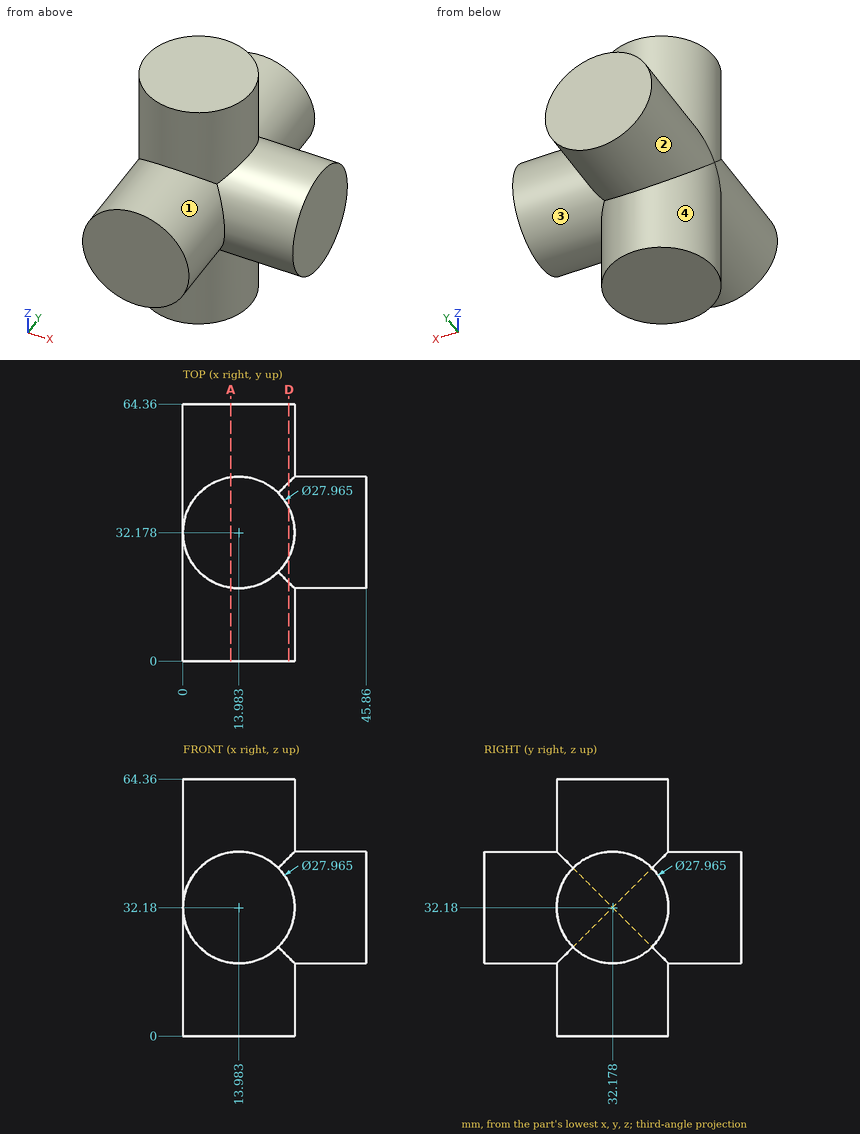
For this review, use the dimensioned drawing (mm, ordinates from the lowest corner) and the shaded views. A direction names the side the tool comes from. Give positions to 0.01 mm unless a question says otherwise; leave off trailing zeros. Order: outer loops, then holes, each group sorted by start corner. A loop starts at its lowest first (then second) coordinate and runs counter-clockwise, first axis right, second up. Notation, with made-up numbers: (78, -25) -> (85, -25) arc R20 ccw to (85, -1) -> close; hole circle Ø2 at (57, 40). An arc over 180 degrees is marked (long way). Write item = value, one per line. Start each with the question number.
(1) Take a section at A-A (x = 12). Write out the cut boundary in (y, z).
(2) For L1, parallel to Y at x = 20, z = 5 (1 decimal); L2, parallel to Z at x = 3, y = 45 (1 decimal); L3, parallel to X at y = 27, z = 27 (1 decimal), list the stretches that pass through material, from the lowest coordinate up. Write a range as from..to.
(3) Take a section at D-D (x = 26.5). Write out the cut boundary in (y, z) (1 decimal).
(4) For pin 1 Ø3 at (x, y) = (13.5, 40) entering from -Z; pin 2 Ø2 at (x, z) = (17, 50.5) entering from -Y; pin 3 Ø1 at (x, y) = (28.5, 34.5) entering from +Z; pin 4 Ø2 at (x, y) = (26.5, 50) entering from +Z, all flat-tipped, find the tip position at first contact; note any pin that passes through.
(5) Tool access review of the marked faces 1, 2, 3 and 4: name each direction out of +Z, -Z, +X, -X, +Y, -Y from which nothing blocks a thin tool from reaching the whole face with its end or side.
Returned:
q1.outline = (0, 18.34) -> (18.34, 18.34) -> (18.34, 0) -> (46.02, 0) -> (46.02, 18.34) -> (64.36, 18.34) -> (64.36, 46.02) -> (46.02, 46.02) -> (46.02, 64.36) -> (18.34, 64.36) -> (18.34, 46.02) -> (0, 46.02) -> close
q2.L1 = 19.6..44.8
q2.L2 = 23.5..40.8
q2.L3 = 1..45.9
q3.outline = (0, 25.9) -> (19.7, 25.9) arc R14 ccw to (25.9, 19.7) -> (25.9, 0) -> (38.4, 0) -> (38.4, 19.7) arc R14 ccw to (44.7, 25.9) -> (64.4, 25.9) -> (64.4, 38.4) -> (44.7, 38.4) arc R14 ccw to (38.4, 44.7) -> (38.4, 64.4) -> (25.9, 64.4) -> (25.9, 44.7) arc R14 ccw to (19.7, 38.4) -> (0, 38.4) -> close
q4.pin_1 = 0
q4.pin_2 = 18.34
q4.pin_3 = 46.04
q4.pin_4 = 40.11
q5.face_1 = -Y
q5.face_2 = +Y
q5.face_3 = +X
q5.face_4 = -Z
